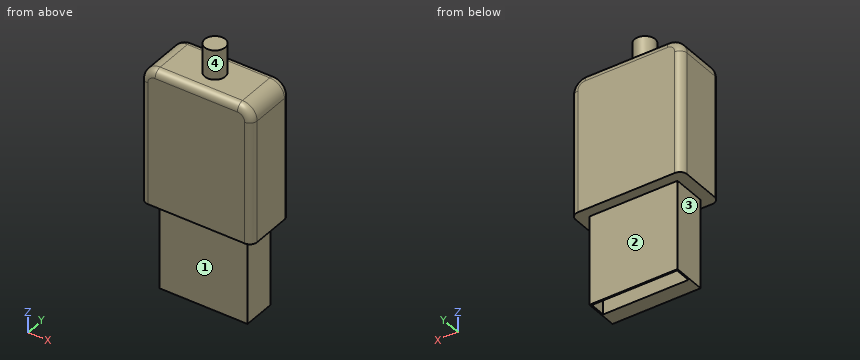
from build123d import *
from OCP.BRepFilletAPI import BRepFilletAPI_MakeFillet

# Parameters (mm, degrees)
ESQUISSE1_W             = 15.2
ESQUISSE1_H             = 7.3
BOSS_EXTRU_1_DEPTH      = 18.6
ESQUISSE2_W             = 12
ESQUISSE2_H             = 4.5
BOSS_EXTRU_2_DEPTH      = 12.1
ESQUISSE3_W             = 11.6
ESQUISSE3_H             = 2.2
ENL_V_MAT_EXTRU_1_DEPTH = 9
ESQUISSE4_R             = 1.4
BOSS_EXTRU_3_DEPTH      = 4
CONG_1_R1               = 1
CONG_1_R2               = 2


with BuildPart() as part:
    # Esquisse1 → Boss.-Extru.1 (new body)
    with BuildSketch(Plane.XY):
        Rectangle(ESQUISSE1_W, ESQUISSE1_H)
    extrude(amount=BOSS_EXTRU_1_DEPTH)

    # Esquisse2 → Boss.-Extru.2 (add)
    with BuildSketch(Plane(origin=(0, 0, 0), x_dir=(-1, 0, 0), z_dir=(0, 0, -1))):
        Rectangle(ESQUISSE2_W, ESQUISSE2_H)
    extrude(amount=BOSS_EXTRU_2_DEPTH)

    # Esquisse3 → Enlèv. mat.-Extru.1 (cut)
    with BuildSketch(Plane(origin=(0, 0, -12.1), x_dir=(-1, 0, 0), z_dir=(0, 0, -1))):
        with Locations((0, 0.95)):
            Rectangle(ESQUISSE3_W, ESQUISSE3_H)
    extrude(amount=-ENL_V_MAT_EXTRU_1_DEPTH, mode=Mode.SUBTRACT)

    # Esquisse4 → Boss.-Extru.3 (add)
    with BuildSketch(Plane.XY.offset(18.6)):
        Circle(ESQUISSE4_R)
    extrude(amount=BOSS_EXTRU_3_DEPTH)

    # Congé1: one fillet with a radius per group of edges: ONE call of the kernel's fillet builder (fillet() takes one radius for all edges)
    cong_1_edges_1 = [part.edges().sort_by_distance(p)[0] for p in [
        (-7.6, 3.65, 9.3),
        (7.6, 3.65, 9.3),
        (7.6, -3.65, 9.3),
        (-7.6, -3.65, 9.3),
        (0, -3.65, 18.6),
        (0, 3.65, 18.6),
    ]]
    cong_1_edges_2 = [part.edges().sort_by_distance(p)[0] for p in [
        (-7.6, 0, 18.6),
        (7.6, 0, 18.6),
    ]]
    cong_1 = BRepFilletAPI_MakeFillet(part.part.solid().wrapped)
    for e in cong_1_edges_1:
        cong_1.Add(CONG_1_R1, e.wrapped)
    for e in cong_1_edges_2:
        cong_1.Add(CONG_1_R2, e.wrapped)
    add(Compound.cast(cong_1.Shape()), mode=Mode.REPLACE)


solid = part.part
Part model, mm, in its own coordinate system. Face numbers are marked on the shaded views. A direction names the side the tool comes from. Give positions to 0.01 mm unless a question says otherwise; leave off trailing zeros. Loops run counter-clockwise (first coordinate to the right, second up) from the corner with the lowest first, then second, coordinate; pieces in that order, holes last. Notation, with made-up numbers: M 18.5,89.5 L 45.5,89.5 A30 ccw 45.5,111.5 Z; hole C -25,36 d9. An arc over 180 degrees is marked long. Put each result on its own line as item: value. Start each with the question number.
1) Saw through at A-A (z = -7). List the corners of the cut face in (x, y).
2) Flat gauge pins, fed straight in: pin 1 (2.5 mm diameter, centred on x = 2.5, z = -7, fed in from +Y); pin 2 (2 mm diameter, centred on y = 1, z = -4.5, fed in from -X); pin 3 (1.6 mm diameter, centred on x = 2.5, y = 0.5, fed in from +Z). Where does each tip first touch, or does it go through?
3) Saw through at B-B (x = -3.5). List the corners of the cut face in (y, z), then the cut area to 3 significant figures.
4) 3-axis set-ups, long thin cutter, end or side, ignore diameter. For the marked faces 1, 2, 3 and 4: which of +Z, -Z, +X, -X, +Y, -Y reach the whole face in a straight line?
5) Saw through at D-D (x = 0). List the corners of the cut face in (y, z).
6) Probe probe 1 along Y at (x, z) = (1.5, -9); probe 2 along X at (y, z) = (-2.75, 8.5); probe 3 along Z at (x, y) = (-0.75, 0). List the from-to ranges inside material, lowest first.
7) Saw through at C-C (y = -1.75). List the corners of the cut face in (x, z).
Numbers:
1. outline: M -6,-2.25 L 6,-2.25 L 6,2.25 L -6,2.25 Z; hole M -5.8,-0.15 L 5.8,-0.15 L 5.8,2.05 L -5.8,2.05 Z
2. pin 1: y = 2.25
2. pin 2: x = -6
2. pin 3: z = 18.6
3. outline: M -3.65,0 L -2.25,0 L -2.25,-12.1 L -0.15,-12.1 L -0.15,-3.1 L 2.05,-3.1 L 2.05,-12.1 L 2.25,-12.1 L 2.25,0 L 3.65,0 L 3.65,17.6 A1 ccw 2.65,18.6 L -2.65,18.6 A1 ccw -3.65,17.6 Z
3. area: 170 mm^2
4. face 1: -Z, +X, -X, -Y
4. face 2: -Z, +X, -X, +Y
4. face 3: -Z, -X, +Y, -Y
4. face 4: +Z
5. outline: M -3.65,0 L -2.25,0 L -2.25,-12.1 L -0.15,-12.1 L -0.15,-3.1 L 2.05,-3.1 L 2.05,-12.1 L 2.25,-12.1 L 2.25,0 L 3.65,0 L 3.65,17.6 A1 ccw 2.65,18.6 L 1.4,18.6 L 1.4,22.6 L -1.4,22.6 L -1.4,18.6 L -2.65,18.6 A1 ccw -3.65,17.6 Z
6. probe 1: -2.25 to -0.15, 2.05 to 2.25
6. probe 2: -7.59 to 7.59
6. probe 3: -3.1 to 22.6
7. outline: M -7.6,0 L -6,0 L -6,-12.1 L 6,-12.1 L 6,0 L 7.6,0 L 7.6,16.6 A2 ccw 5.6,18.6 L -5.6,18.6 A2 ccw -7.6,16.6 Z
